Can you work these out from the model? Positions are in its coordinate system, mm. Round coordinates to 2 decimals unless told otherwise and drop trailing zeros. Loops run counter-clockwise (first coordinate to the right, second up) from the corner with the lowest first, then second, coordinate; pieces in that order, holes last. Notation, with made-up numbers: (-34.5, -8) -> (22.5, -8) arc R8 ccw to (22.5, 7) -> close; hole circle Ø11 at (15.5, -32). An arc over 180 degrees is marked (long way). Answer as a JSON object with one key per item and string values.
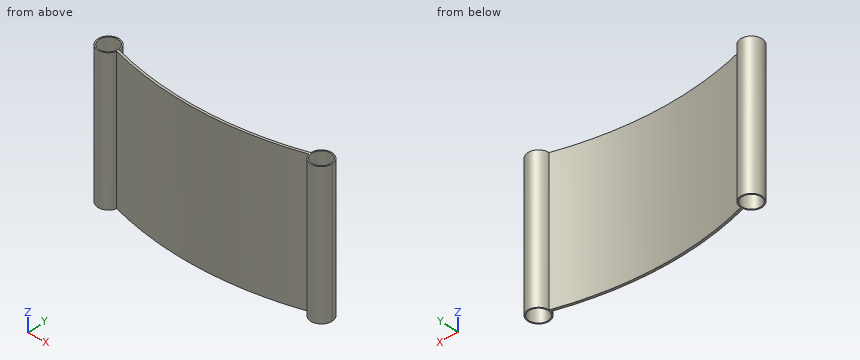
```python
from build123d import *

# Parameters (mm, degrees)
SKETCH2_R             = 4.5
SKETCH2_R_2           = 4
BOSS_EXTRUDE1_DEPTH   = 60
BOSS_EXTRUDE1_2_DEPTH = 60
BOSS_EXTRUDE2_DEPTH   = 60


with BuildPart() as part:
    # Sketch2 → Boss-Extrude1 (new body)
    with BuildSketch(Plane.XY):
        with Locations((-45, 0)):
            Circle(SKETCH2_R)
        with Locations((-45, 0)):
            Circle(SKETCH2_R_2, mode=Mode.SUBTRACT)
    extrude(amount=-BOSS_EXTRUDE1_DEPTH)



with BuildPart() as body_2:
    # Sketch2 → Boss-Extrude1 2 (new body)
    with BuildSketch(Plane.XY):
        with Locations((45, 0)):
            Circle(SKETCH2_R)
        with Locations((45, 0)):
            Circle(SKETCH2_R_2, mode=Mode.SUBTRACT)
    extrude(amount=-BOSS_EXTRUDE1_2_DEPTH)


with BuildPart() as part_1:
    add(part.part)

    add(body_2.part)  # Boss-Extrude2 merges body 2
    # Sketch3 → Boss-Extrude2 (add)
    with BuildSketch(Plane.XY):
        with BuildLine():
            Line((40.5, 0), (40.793767043, -0.955877045))
            ThreePointArc((40.793767043, -0.955877045), (0, -7.082982188), (-40.793767043, -0.955877045))
            Line((-40.793767043, -0.955877045), (-40.5, 0))
            ThreePointArc((-40.5, 0), (0, -6.082982188), (40.5, 0))
        make_face()
    extrude(amount=-BOSS_EXTRUDE2_DEPTH)


solid = part_1.part
```
Q1. I want a section at A-A, the plane x = 45. Write out the boundary of the cut face in (y, z), then the cut area to 3 significant figures.
Determined:
{"outline": "(-4.5, -60) -> (-4, -60) -> (-4, 0) -> (-4.5, 0) -> close; (4, -60) -> (4.5, -60) -> (4.5, 0) -> (4, 0) -> close", "area": "60.0 mm²"}
Q2. I'm going to push flat-ended pins straight in: pin 1 (4 mm diameter, centred on y = -4, z = -9, fed in from +X); pin 2 (6 mm diameter, centred on x = 16.5, z = -44, fed in from -Y); pin 3 (5 mm diameter, centred on x = -11, z = -24, fed in from +Y). Where does each tip first touch, or does it pass through?
Determined:
{"pin 1": "x = 49.03", "pin 2": "y = -6.43", "pin 3": "y = -5.42"}
Q3. I want a section at B-B, the plane z = -46.5. Write out the boundary of the cut face in (x, y), then the cut area to 3 significant figures.
Determined:
{"outline": "(-40.61, -1.01) arc R138.86 ccw to (40.61, -1.01) arc R4.5 ccw (long way) to (40.5, 0) arc R137.86 cw to (-40.5, 0) arc R4.5 ccw (long way) to start; hole circle Ø8 at (-45, 0); hole circle Ø8 at (45, 0)", "area": "109 mm²"}
Q4. If I drill on L1, parallel to Y at x = 45, z = -47; L2, parallel to X at y = 0.75, z = -32; L3, parallel to Y at x = -1, z = -10, over which ranges is the centre line in solid material (lowest first)? Write a range as [from, to].
Determined:
{"L1": "[-4.5, -4], [4, 4.5]", "L2": "[-49.44, -48.93], [-41.07, -40.56], [40.56, 41.07], [48.93, 49.44]", "L3": "[-7.08, -6.08]"}
Q5. I want a section at C-C, the plane x = 11.5. Write out the boundary of the cut face in (y, z), then the cut area to 3 significant figures.
Determined:
{"outline": "(-6.61, -60) -> (-5.6, -60) -> (-5.6, 0) -> (-6.61, 0) -> close", "area": "60.2 mm²"}
Q6. I want a section at D-D, the plane x = 22. Write out the boundary of the cut face in (y, z).
Determined:
{"outline": "(-5.33, -60) -> (-4.32, -60) -> (-4.32, 0) -> (-5.33, 0) -> close"}
